```python
from build123d import *

# Parameters (mm, degrees)
F0_R     = 16.4
F0_R_2   = 11.5
F1_DEPTH = 1.2
F0_R_3   = 10
F2_DEPTH = 3
F3_R     = 1.500919
F4_DEPTH = 25


with BuildPart() as f1:
    # F0 (on Top) → F1 (new body)
    with BuildSketch(Plane.XY):
        with Locations((-45.598116, 14.504182)):
            Circle(F0_R)
        with Locations((-45.598116, 14.504182)):
            Circle(F0_R_2, mode=Mode.SUBTRACT)
    extrude(amount=F1_DEPTH)

    # F0 (on Top) → F2 (join)
    with BuildSketch(Plane.XY):
        with Locations((-45.598116, 14.504182)):
            Circle(F0_R_2)
        with Locations((-45.598116, 14.504182)):
            Circle(F0_R_3, mode=Mode.SUBTRACT)
    extrude(amount=F2_DEPTH)

    # F3 (on face) → F4 (cut)
    with BuildSketch(Plane.XY.offset(1.2)):
        with Locations((-45.598116, 27.51958)):
            Circle(F3_R)
        with Locations((-49.620095, 26.882561)):
            Circle(F3_R)
        with Locations((-53.248375, 25.03386)):
            Circle(F3_R)
        with Locations((-56.127794, 22.154441)):
            Circle(F3_R)
        with Locations((-57.976495, 18.526161)):
            Circle(F3_R)
        with Locations((-58.613514, 14.504182)):
            Circle(F3_R)
        with Locations((-57.976495, 10.482203)):
            Circle(F3_R)
        with Locations((-56.127794, 6.853923)):
            Circle(F3_R)
        with Locations((-53.248375, 3.974504)):
            Circle(F3_R)
        with Locations((-49.620095, 2.125803)):
            Circle(F3_R)
        with Locations((-45.598116, 1.488784)):
            Circle(F3_R)
        with Locations((-41.576137, 2.125803)):
            Circle(F3_R)
        with Locations((-37.947857, 3.974504)):
            Circle(F3_R)
        with Locations((-35.068438, 6.853923)):
            Circle(F3_R)
        with Locations((-33.219737, 10.482203)):
            Circle(F3_R)
        with Locations((-32.582718, 14.504182)):
            Circle(F3_R)
        with Locations((-33.219737, 18.526161)):
            Circle(F3_R)
        with Locations((-35.068438, 22.154441)):
            Circle(F3_R)
        with Locations((-37.947857, 25.03386)):
            Circle(F3_R)
        with Locations((-41.576137, 26.882561)):
            Circle(F3_R)
    extrude(amount=-F4_DEPTH, mode=Mode.SUBTRACT)


solid = f1.part
```
Geometry: final body of the model. Coordinates: model frame, mm. A direction names the side the tool comes from. Round coordinates to 2 decimals unless told otherwise and drop trailing zeros. Loops run counter-clockwise (first coordinate to the right, second up) from the corner with the lowest first, then second, coordinate; pieces in that order, holes last.
Item 1: Line query: L1, parallel to X at y = 7, z = 0.25; L2, parallel to X at y = 14, z = 0.45; L3, parallel to Y at x = -57, z = 0.95. Output: solid intervals per line, ascending.
Checked values:
L1: x = -60.18 to -57.62, -54.63 to -52.21, -38.99 to -36.56, -33.57 to -31.02
L2: x = -61.99 to -60.03, -57.2 to -55.59, -35.61 to -34, -31.17 to -29.21
L3: y = 2.72 to 5.63, 8.08 to 9.34, 11.62 to 17.39, 19.67 to 20.93, 23.38 to 26.29
Item 2: Contact query for flat-ended pins moving along their axis: P1, Ø1, axis at y = 7.5, z = 1.5, coming from the -X side; P2, Ø1, axis at y = 20.5, z = 1, coming from the +X side; P3, Ø1.5, axis at x = -50, z = 2, coming from the +Y side. Output: stop coordinate, or through.
Checked values:
P1: stops at x = -60.61
P2: stops at x = -30.15
P3: stops at y = 25.41
Item 3: Section D-D, the plane z = 2.3. Output: boundary loops of the cut face in (x, y).
Checked values:
outline: circle Ø23 at (-45.6, 14.5); hole circle Ø20 at (-45.6, 14.5)
Item 4: Mould query, pull axis X, two halves, no side actions, for faces 3 (the cylindrical face through (-47.733, 30.765, 0.592)), 4 (the flat face through (-46, 25, 3)), 5 (the cylindrical face through (-59.17, 9.57, 0.61)). Classes: released by +X, released by -X, zero draft, split by the parting line, or undercut.
Checked values:
face 3: split by the parting line
face 4: zero draft
face 5: undercut
Item 5: Section B-B, the plane x = -39. Output: boundary loops of the cut face in (y, z).
Checked values:
outline: (-0.51, 0) - (2.9, 0) - (2.9, 1.2) - (-0.51, 1.2) - close; (5.04, 0) - (6.99, 0) - (6.99, 3) - (5.09, 3) - (5.09, 1.2) - (5.04, 1.2) - close; (22.02, 0) - (23.96, 0) - (23.96, 1.2) - (23.92, 1.2) - (23.92, 3) - (22.02, 3) - close; (26.1, 0) - (29.52, 0) - (29.52, 1.2) - (26.1, 1.2) - close
Item 6: Section C-C, the plane z = 0.5. State how many separate pieces and enclosed holes the cut face has, plus the area to 3 significant figures.
Checked values:
separate pieces: 1
enclosed holes: 21
area: 389 mm2
Item 7: Reachability of faces 1 (the flat face through (-38, 7, 0)), 2 (the cylindrical face through (-34.975, 10.1, 2.087)) from +Z, -Z, +X, -X, +Y, -Y: full face, straight path, thin tool, end or side. Return the list, or none.
Checked values:
face 1: -Z, +X, -X, +Y, -Y
face 2: +Z
Item 8: Section A-A, the plane y = 15. Output: boundary loops of the cut face in (x, z), plus the area to 3 significant figures.
Checked values:
outline: (-61.99, 0) - (-60.03, 0) - (-60.03, 1.2) - (-61.99, 1.2) - close; (-57.2, 0) - (-55.59, 0) - (-55.59, 3) - (-57.09, 3) - (-57.09, 1.2) - (-57.2, 1.2) - close; (-35.61, 0) - (-34, 0) - (-34, 1.2) - (-34.11, 1.2) - (-34.11, 3) - (-35.61, 3) - close; (-31.17, 0) - (-29.21, 0) - (-29.21, 1.2) - (-31.17, 1.2) - close
area: 14.0 mm2
